Verification items for the finished model (mm, model axes). A direction names the side the tool comes from. Round coordinates to 2 decimals unless told otherwise and drop trailing zeros. Write each loop counter-clockwise with the first axis right and the second up, starting at its lowest first coordinate (ties: lowest second). Pieces come first, ordered by that corner, then holes. Notation, with made-up numbers: (76, 11.5) -> (85, 11.5) arc R16 ccw to (85, 21.5) -> close; hole circle Ø6 at (-24.75, 3.25). An arc over 180 degrees is marked (long way). Answer as a JSON object with one key per item and string values. Group by question number.
(1) Scan lines: L1, parallel to X at y = -0.05, z = 12.5; L2, parallel to Z at x = -2.2, y = 0.35; L3, parallel to Z at x = -1.6, y = 2.1. Record each from-to range of solid material in increasing order. Write a range as from..to.
(2) Sectioned sample at C-C on y = 0. Record the cut outline in (x, z) (3 decimals).
(3) Sectioned sample at B-B on z = 32. Record the cut outline in (x, y) (3 decimals), and give its area (3 significant figures).
(4) Sectioned sample at D-D on z = 20. Record the cut outline in (x, y), and give its area (3 significant figures).
(5) Set-up check for faces 4 (the face through (0.2, -2.2, 38.8)), 5 (the face through (0, 1.85, 35)), 6 (the face through (1.874, 0.699, 14.198)): record each of +Z, -Z, +X, -X, +Y, -Y from which the full face is reachable in a straight line by a thin tool's end or side.
(6) Draft check along X on faces 1 (the face through (0, 0, 0)), 2 (the face through (2.725, -0.028, 34.856)), 3 (the face through (0.02, 2.35, 9.44)). Enter one of: released by +X, released by -X, zero draft, split by the parting line, or undercut.
(7) Gauge pin test, flat ends, axial feed: pin 1 Ø3 at (x, y) = (-0.5, 0) entering from +Z; pin 2 Ø3 at (x, z) = (0.5, 11.5) entering from +Y; pin 3 Ø1.5 at (x, z) = (2, 5) entering from -Y. Record the tip position at first contact, or that the pin passes through.
(8) Sectioned sample at A-A on x = 0. Record the cut outline in (y, z).
```python
from build123d import *

# Parameters (mm, degrees)
SKETCH3_R           = 2
BOSS_EXTRUDE1_DEPTH = 5.2
SKETCH4_R           = 2
BOSS_EXTRUDE2_DEPTH = 8.6
SKETCH5_R           = 2
BOSS_EXTRUDE3_DEPTH = 15
SKETCH6_R           = 3
BOSS_EXTRUDE4_DEPTH = 10
CUT_EXTRUDE1_DEPTH  = 8


with BuildPart() as part:
    # Sketch3 → Boss-Extrude1 (new body)
    with BuildSketch(Plane.XY):
        Circle(SKETCH3_R)
    extrude(amount=BOSS_EXTRUDE1_DEPTH)

    # Sketch4 → Boss-Extrude2 (add)
    with BuildSketch(Plane.XY.offset(5.2)):
        with Locations(Location((0, 0, 0), (0, 0, 119))):
            Circle(SKETCH4_R)
        with BuildLine():
            Line((0, 0), (1.139302608, 2.055356312))
            ThreePointArc((1.139302608, 2.055356312), (0, 2.35), (-1.139302608, 2.055356312))
            Line((-1.139302608, 2.055356312), (0, 0))
        make_face()
        with BuildLine():
            Line((0.96961924, 1.749239414), (0, 0))
            Line((0, 0), (-0.96961924, 1.749239414))
            ThreePointArc((-0.96961924, 1.749239414), (-1.015076726, -1.723258321), (2, 0))
            ThreePointArc((2, 0), (1.723258321, 1.015076726), (0.96961924, 1.749239414))
        make_face()
    extrude(amount=BOSS_EXTRUDE2_DEPTH)

    # Sketch5 → Boss-Extrude3 (add)
    with BuildSketch(Plane.XY.offset(13.8)):
        Circle(SKETCH5_R)
    extrude(amount=BOSS_EXTRUDE3_DEPTH)

    # Sketch6 → Boss-Extrude4 (add)
    with BuildSketch(Plane.XY.offset(28.8)):
        Circle(SKETCH6_R)
    extrude(amount=BOSS_EXTRUDE4_DEPTH)

    # Sketch7 → Cut-Extrude1 (cut)
    with BuildSketch(Plane.XY.offset(38.8)):
        with BuildLine():
            Line((2.000781097, 1.85), (-2.000781097, 1.85))
            ThreePointArc((-2.000781097, 1.85), (-2.725, 0), (-2.000781097, -1.85))
            Line((-2.000781097, -1.85), (2.000781097, -1.85))
            ThreePointArc((2.000781097, -1.85), (2.725, 0), (2.000781097, 1.85))
        make_face()
    extrude(amount=-CUT_EXTRUDE1_DEPTH, mode=Mode.SUBTRACT)


solid = part.part
```
Computed values:
{
 "1": {"L1": "-2..2", "L2": "28.8..30.8", "L3": "28.8..38.8"},
 "2": {"outline": "(-3, 28.8) -> (-2, 28.8) -> (-2, 0) -> (2, 0) -> (2, 28.8) -> (3, 28.8) -> (3, 38.8) -> (2.725, 38.8) -> (2.725, 30.8) -> (-2.725, 30.8) -> (-2.725, 38.8) -> (-3, 38.8) -> close"},
 "3": {"outline": "circle Ø6 at (0, 0); hole (-2.001, -1.85) -> (2.001, -1.85) arc R2.725 ccw to (2.001, 1.85) -> (-2.001, 1.85) arc R2.725 ccw to start", "area": "9.79 mm2"},
 "4": {"outline": "circle Ø4 at (0, 0)", "area": "12.6 mm2"},
 "5": {"face 4": "+Z, +X, -X, +Y, -Y", "face 5": "+Z", "face 6": "none"},
 "6": {"face 1": "zero draft", "face 2": "undercut", "face 3": "split by the parting line"},
 "7": {"pin 1": "z = 30.8", "pin 2": "y = 2.35", "pin 3": "y = -1.56"},
 "8": {"outline": "(-3, 28.8) -> (-2, 28.8) -> (-2, 0) -> (2, 0) -> (2, 5.2) -> (2.35, 5.2) -> (2.35, 13.8) -> (2, 13.8) -> (2, 28.8) -> (3, 28.8) -> (3, 38.8) -> (1.85, 38.8) -> (1.85, 30.8) -> (-1.85, 30.8) -> (-1.85, 38.8) -> (-3, 38.8) -> close"}
}
